Geometry check sheet. Reference: the model listing, model coordinates, mm. Round coordinates to 2 decimals unless told otherwise and drop trailing zeros. Loops run counter-clockwise (first coordinate to the right, second up) from the corner with the lowest first, then second, coordinate; pieces in that order, holes last.
```python
from build123d import *

# Parameters (mm, degrees)
SKETCH1_R           = 64.5
SKETCH1_R_2         = 1.65
SKETCH1_R_3         = 13
SKETCH1_R_4         = 1.4
BOSS_EXTRUDE2_DEPTH = 3.175
SKETCH2_W           = 3.175
SKETCH2_H           = 8
CUT_EXTRUDE1_DEPTH  = 4.175
SKETCH3_W           = 31
SKETCH3_H           = 55
CUT_EXTRUDE2_DEPTH  = 4.175
FILLET3_R           = 1


with BuildPart() as part:
    # Sketch1 → Boss-Extrude2 (new body)
    with BuildSketch(Plane(origin=(0, 0, 0), x_dir=(-1, 0, 0), z_dir=(0, 0, 1))):
        with Locations((14.45539036, 0.366425758)):
            Circle(SKETCH1_R)
        with Locations((26.018596538, -38.058574242)):
            Circle(SKETCH1_R_2, mode=Mode.SUBTRACT)
        with Locations((4.318596538, -38.058574242)):
            Circle(SKETCH1_R_2, mode=Mode.SUBTRACT)
        with Locations((26.018596538, 38.791425758)):
            Circle(SKETCH1_R_2, mode=Mode.SUBTRACT)
        with Locations((4.318596538, 38.791425758)):
            Circle(SKETCH1_R_2, mode=Mode.SUBTRACT)
        with Locations((14.45539036, 0.366425758)):
            Circle(SKETCH1_R_3, mode=Mode.SUBTRACT)
        with Locations((-6.54460964, 56.366425758)):
            Circle(SKETCH1_R_2, mode=Mode.SUBTRACT)
        with Locations((-22.394874657, 46.366425758)):
            Circle(SKETCH1_R_2, mode=Mode.SUBTRACT)
        with Locations((35.45539036, 56.366425758)):
            Circle(SKETCH1_R_2, mode=Mode.SUBTRACT)
        with Locations((51.305655378, 46.366425758)):
            Circle(SKETCH1_R_2, mode=Mode.SUBTRACT)
        with Locations((51.305655378, -45.633574242)):
            Circle(SKETCH1_R_2, mode=Mode.SUBTRACT)
        with Locations((35.45539036, -55.633574242)):
            Circle(SKETCH1_R_2, mode=Mode.SUBTRACT)
        with Locations((-6.54460964, -55.633574242)):
            Circle(SKETCH1_R_2, mode=Mode.SUBTRACT)
        with Locations((-22.394874657, -45.633574242)):
            Circle(SKETCH1_R_2, mode=Mode.SUBTRACT)
        with Locations((18.66683861, -38.633574242)):
            Circle(SKETCH1_R_4, mode=Mode.SUBTRACT)
        with Locations((-30.33316139, -38.633574242)):
            Circle(SKETCH1_R_4, mode=Mode.SUBTRACT)
        with Locations((18.66683861, 19.366425758)):
            Circle(SKETCH1_R_4, mode=Mode.SUBTRACT)
        with Locations((-30.33316139, 19.366425758)):
            Circle(SKETCH1_R_4, mode=Mode.SUBTRACT)
    extrude(amount=BOSS_EXTRUDE2_DEPTH)

    # Sketch2 → Cut-Extrude1 (cut, through all)
    with BuildSketch(Plane.XY.offset(3.175)):
        with Locations((33.95710964, -10.366425758)):
            Rectangle(SKETCH2_W, SKETCH2_H)
        with Locations((33.95710964, 9.633574242)):
            Rectangle(SKETCH2_W, SKETCH2_H)
        with Locations((-62.86789036, 9.633574242)):
            Rectangle(SKETCH2_W, SKETCH2_H)
        with Locations((-62.86789036, -10.366425758)):
            Rectangle(SKETCH2_W, SKETCH2_H)
    extrude(amount=-CUT_EXTRUDE1_DEPTH, mode=Mode.SUBTRACT)

    # Sketch3 → Cut-Extrude2 (cut, through all)
    with BuildSketch(Plane.XY.offset(3.175)):
        with Locations((-39.95539036, -0.366425758)):
            Rectangle(SKETCH3_W, SKETCH3_H)
    extrude(amount=-CUT_EXTRUDE2_DEPTH, mode=Mode.SUBTRACT)

    # Fillet3
    fillet3_edges = [part.edges().sort_by_distance(p)[0] for p in [
        (-24.45539036, 7.940198105, 1.5875),
        (-24.45539036, -8.673049621, 1.5875),
    ]]
    fillet(fillet3_edges, radius=FILLET3_R)


solid = part.part
```
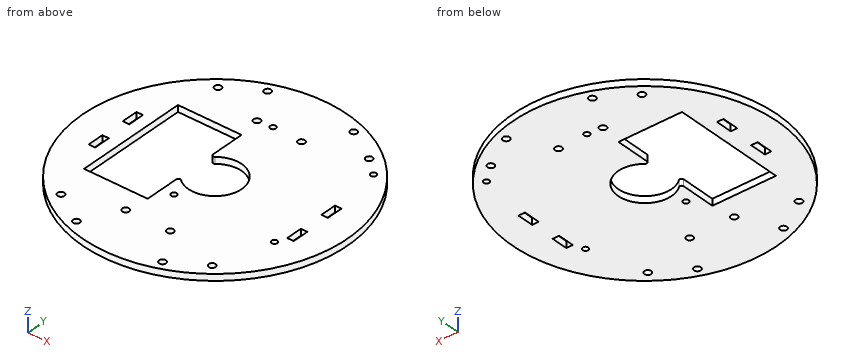
1) Sectioned sample at D-D, the plane z = 2.5. State how many separate pieces and enclosed holes the cut face has, then the cut area to 3 significant figures.
Report:
separate pieces: 1
enclosed holes: 21
area: 10,600 mm2
2) Sectioned sample at A-A, the plane y = -25.5. Record the cut outline in (x, z) (3 decimals).
Report:
outline: (-73.857, 0) - (-55.455, 0) - (-55.455, 3.175) - (-73.857, 3.175) - close; (-24.455, 0) - (44.946, 0) - (44.946, 3.175) - (-24.455, 3.175) - close
3) Scan lines: line 1 along Y through (x, z) = (-35.5, 1.2); line 2 along X through (y, z) = (-46.5, 2.6); line 3 along X through (y, z) = (-46, 2.8). Record each from-to range of solid material in increasing order.
Report:
line 1: y = -61.34 to -58.02, -54.72 to -27.87, 27.13 to 53.98, 57.28 to 60.6
line 2: x = -59.53 to -52.95, -49.66 to 20.75, 24.04 to 30.62
line 3: x = -60.04 to -52.91, -49.7 to 20.79, 24 to 31.13
4) Sectioned sample at B-B, the plane x = -45. Record the cut outline in (y, z) (3 decimals).
Report:
outline: (-57.176, 0) - (-27.866, 0) - (-27.866, 3.175) - (-57.176, 3.175) - close; (27.134, 0) - (56.443, 0) - (56.443, 3.175) - (27.134, 3.175) - close
5) Sectioned sample at C-C, the plane y = -8. Record the cut outline in (x, z) (3 decimals), then the cut area to 3 significant figures.
Report:
outline: (-78.502, 0) - (-64.455, 0) - (-64.455, 3.175) - (-78.502, 3.175) - close; (-61.28, 0) - (-55.455, 0) - (-55.455, 3.175) - (-61.28, 3.175) - close; (-3.933, 0) - (32.37, 0) - (32.37, 3.175) - (-3.933, 3.175) - close; (35.545, 0) - (49.591, 0) - (49.591, 3.175) - (35.545, 3.175) - close
area: 223 mm2
6) Gauge pin test, flat ends, axial feed: pin 1 (1.6 mm diameter, centred on x = -62.5, z = 1, fed in from +Y); pin 2 (3 mm diameter, centred on x = -4.32, y = -38.79, fed in from +Z); pin 3 (1 mm diameter, centred on x = -42.5, y = 50, fed in from -Z); pin 4 (1.6 mm diameter, centred on y = 8.5, z = 1.5, fed in from -X). Record the tip position at first contact, or that the pin passes through.
Report:
pin 1: stops at y = 43.54
pin 2: passes through
pin 3: stops at z = 0
pin 4: stops at x = -78.45
